from build123d import *

# Parameters (mm, degrees)
F0_R     = 15
F1_DEPTH = 3
F3_DEPTH = 20
F4_R     = 9
F4_R_2   = 7.5
F5_DEPTH = 18
F7_DEPTH = 3
F9_DEPTH = 40


with BuildPart() as f1:
    # F0 (on Top) → F1 (new body)
    with BuildSketch(Plane.XY):
        Circle(F0_R)
    extrude(amount=F1_DEPTH)

    # F2 (on Front) → F3 (cut, symmetric)
    with BuildSketch(Plane.XZ):
        Polygon((-16.27984, 1.543784), (0, 2.968085), (16.030641, 1.565586), (16.030641, 3.755485), (-16.27984, 3.755485), align=None)
    extrude(amount=F3_DEPTH, both=True, mode=Mode.SUBTRACT)

    # F4 (on Top) → F5 (join)
    with BuildSketch(Plane.XY):
        Circle(F4_R)
        Circle(F4_R_2, mode=Mode.SUBTRACT)
    extrude(amount=F5_DEPTH)

    # F6 (on Front) → F7 (cut, symmetric)
    with BuildSketch(Plane.XZ):
        Polygon((16.263659, 20.495596), (-16.880802, 20.495596), (-16.596312, 1.516096), (0, 2.968085), (16.263659, 1.545199), align=None)
    extrude(amount=F7_DEPTH, both=True, mode=Mode.SUBTRACT)

    # F8 (on face) → F9 (join)
    with BuildSketch(Plane.XY.offset(18)):
        with BuildLine():
            Line((6.873864, 3), (8.485281, 3))
            ThreePointArc((8.485281, 3), (0, 9), (-8.485281, 3))
            Line((-8.485281, 3), (-6.873864, 3))
            ThreePointArc((-6.873864, 3), (0, 7.5), (6.873864, 3))
        make_face()
    extrude(amount=F9_DEPTH)


solid = f1.part
Verification items for the finished model (mm, model axes). A direction names the side the tool comes from. Coordinates: 2 decimals unless noted, no trailing zeros. Order: outer loops, then holes, each group sorted by start corner. A loop starts at its lowest first (then second) coordinate and runs counter-clockwise, first axis right, second up.
1. Sectioned sample at B-B, the plane y = 0. Record the cut outline in (x, z).
Results found:
outline: (-15, 0) - (15, 0) - (15, 1.66) - (0, 2.97) - (-15, 1.66) - close
2. Set-up check for faces 4 (the face through (-0.1, -7.5, 10.1)), 5 (the face through (0, -9, 10)), 6 (the face through (0, 8, 58)): record each of +Z, -Z, +X, -X, +Y, -Y from which the full face is reachable in a straight line by a thin tool's end or side.
Results found:
face 4: +Z
face 5: +Z, -Y
face 6: +Z, +X, -X, +Y, -Y
3. Sectioned sample at D-D, the plane z = 31. Record the cut outline in (x, y), and give its area (3 significant figures).
Results found:
outline: (-8.49, 3) - (-6.87, 3) arc R7.5 cw to (6.87, 3) - (8.49, 3) arc R9 ccw to start
area: 29.7 mm2
4. Release check for a two-part mould opening along Y. For faces 1 (the face through (8, -3, 10)), 2 (the face through (0, -8, 18)), 3 (the face through (-11.056, 10.138, 1.133)) record: +Y half, -Y half, draft (parallel to the pull), parting line (faces both ways), or undercut.
Results found:
face 1: undercut
face 2: draft
face 3: parting line
5. Sectioned sample at C-C, the plane x = -3.5. Record the cut outline in (y, z).
Results found:
outline: (-14.59, 0) - (14.59, 0) - (14.59, 2.66) - (8.29, 2.66) - (8.29, 58) - (6.63, 58) - (6.63, 2.66) - (-6.63, 2.66) - (-6.63, 18) - (-8.29, 18) - (-8.29, 2.66) - (-14.59, 2.66) - close
6. Go/stop test with flat-tipped pins: pin 1 Ø0.8 at (x, z) = (-7.5, 10.5) entering from +Y; pin 2 Ø1.8 at (x, y) = (-3, -6) entering from +Z; pin 3 Ø1.5 at (y, z) = (4.5, 51) entering from -X. Record where each tip stops, or that it passes through.
Results found:
pin 1: stops at y = 5.53
pin 2: stops at z = 18
pin 3: stops at x = -8.18
7. Scan lines: line 1 (Z direction, x = 7, y = 11.75); line 2 (Y direction, x = -1.75, z = 15); line 3 (Y direction, x = -4.5, z = 12.5). Record each from-to range of solid material in increasing order.
Results found:
line 1: z = 0 to 2.36
line 2: y = -8.83 to -7.29, 7.29 to 8.83
line 3: y = -7.79 to -6, 6 to 7.79
8. Sectioned sample at A-A, the plane z = 10.5. Record the cut outline in (x, y), and give its area (3 significant figures).
Results found:
outline: (-8.49, -3) arc R9 ccw to (8.49, -3) - (6.87, -3) arc R7.5 cw to (-6.87, -3) - close; (-8.49, 3) - (-6.87, 3) arc R7.5 cw to (6.87, 3) - (8.49, 3) arc R9 ccw to start
area: 59.3 mm2
